Geometry check sheet. Reference: the model listing, model coordinates, mm. A direction names the side the tool comes from. Coordinates: 2 decimals unless noted, no trailing zeros. Write each loop counter-clockwise with the first axis right and the second up, starting at its lowest first coordinate (ties: lowest second). Pieces come first, ordered by that corner, then holes. Notation, with made-up numbers: (70, -16.75) -> (120, -16.75) arc R27 cw to (120, 9.25) -> close; hole circle Ø8 at (75, 56). An arc over 180 degrees is marked (long way). One line per question, with ' | ' between items.
```python
from build123d import *

# Parameters (mm, degrees)
EXTRUDE_1_DEPTH                = 4
CUT_EXTRUDE_1_DEPTH            = 105.27847333
CUT_EXTRUDE_1_DEPTH_BACK       = 105.27847333
SKETCH_2_R                     = 2
SKETCH_2_W                     = 4
SKETCH_2_H                     = 16
CHAMFER_1_SIZE                 = 1
CUT_EXTRUDE_2_DEPTH            = 105.27847333
CUT_EXTRUDE_2_DEPTH_BACK       = 105.27847333
SKETCH_6_W                     = 20
SKETCH_6_H                     = 5
EXTRUDE_2_DEPTH                = 25
CHAMFER_2_SIZE                 = 1
EXTRUDE_START                  = -5
EXTRUDE_3_DEPTH                = 5
SKETCH_8_R                     = 6
EXTRUDE_4_DEPTH                = 5
CHAMFER_3_SIZE                 = 1
SKETCH_9_R                     = 4
EXTRUDE_5_DEPTH                = 5
CUT_EXTRUDE_START              = -10
SKETCH_10_R                    = 2
CUT_EXTRUDE_3_DEPTH            = 120.608393839
HOLE_WIZARD_1_4_0_15748031_1_D = 3.999999874
SKETCH_13_R                    = 1.5
CUT_EXTRUDE_4_DEPTH            = 109.434311913
SKETCH_14_R                    = 2
CUT_EXTRUDE_5_DEPTH            = 109.434311913
CUT_EXTRUDE_START_2            = 10
SKETCH_15_R                    = 4
CUT_EXTRUDE_6_DEPTH            = 10
CHAMFER_4_SIZE                 = 2
CHAMFER_5_SIZE                 = 1
SKETCH_16_W                    = 18
SKETCH_16_H                    = 4
CUT_EXTRUDE_7_DEPTH            = 109.434311913
SKETCH_17_R                    = 1.5
CUT_EXTRUDE_8_DEPTH            = 3


with BuildPart() as part:
    # 草图1 → 凸台-拉伸1 (new body)
    with BuildSketch(Plane(origin=(0, 0, 0), x_dir=(1, 0, 0), z_dir=(0, 1, 0))):
        Polygon((0, -34), (0, 34), (17, 47), (32, 47), (32, 34), (55, 34), (55, 47), (61, 47), (63, 45), (93, 45), (93, -45), (63, -45), (61, -47), (55, -47), (55, -34), (32, -34), (32, -47), (17, -47), align=None)
    extrude(amount=EXTRUDE_1_DEPTH)

    # 草图2 → 切除-拉伸1 (cut, two sides: drawn at the far end of the back side and taken through both)
    with BuildSketch(Plane(origin=(0, 4, 0), x_dir=(1, 0, 0), z_dir=(0, 1, 0)).offset(-CUT_EXTRUDE_1_DEPTH_BACK)):
        with Locations(Location((13, 10, 0), (0, 0, 270))):
            Circle(SKETCH_2_R)
        with Locations(Location((13, -10, 0), (0, 0, 90))):
            Circle(SKETCH_2_R)
        with Locations((6, 0)):
            Rectangle(SKETCH_2_W, SKETCH_2_H)
        Polygon((4, 12), (4, 26), (17, 36.408329997), (17, 33.205766921), (8, 26), (8, 12), align=None)
        Polygon((8, -26), (8, -12), (4, -12), (4, -26), (17, -36.408329997), (17, -33.205766921), align=None)
    extrude(amount=CUT_EXTRUDE_1_DEPTH + CUT_EXTRUDE_1_DEPTH_BACK, mode=Mode.SUBTRACT)

    # 倒角1
    chamfer_1_edges = [part.edges().sort_by_distance(p)[0] for p in [
        (8.5, 4, 40.5),
        (24.5, 4, 47),
        (8.5, 4, -40.5),
        (24.5, 4, -47),
        (0, 4, 0),
    ]]
    chamfer(chamfer_1_edges, length=CHAMFER_1_SIZE)

    # 草图3 → 切除-拉伸2 (cut, two sides: drawn at the far end of the back side and taken through both)
    with BuildSketch(Plane(origin=(0, 4, 0), x_dir=(1, 0, 0), z_dir=(0, 1, 0)).offset(-CUT_EXTRUDE_2_DEPTH_BACK)):
        Polygon((93, 22), (33, 22), (21, 10), (21, -10), (33, -22), (93, -22), align=None)
    extrude(amount=CUT_EXTRUDE_2_DEPTH + CUT_EXTRUDE_2_DEPTH_BACK, mode=Mode.SUBTRACT)

    # 草图6 → 凸台-拉伸2 (add)
    with BuildSketch(Plane(origin=(0, 4, 0), x_dir=(1, 0, 0), z_dir=(0, 1, 0))):
        with BuildLine():
            Line((21, 10), (21, 15))
            ThreePointArc((21, 15), (15, 21), (21, 27))
            Line((21, 27), (33, 27))
            Line((33, 27), (33, 22))
            Line((33, 22), (21, 10))
        make_face()
        with Locations((83, 24.5)):
            Rectangle(SKETCH_6_W, SKETCH_6_H)
    extrude_2 = extrude(amount=EXTRUDE_2_DEPTH)

    # 镜向1: 凸台-拉伸2 across plane
    add(extrude_2.mirror(Plane.XY))

    # 倒角2
    chamfer_2_edges = [part.edges().sort_by_distance(p)[0] for p in [
        (83, 4, -27),
        (73, 4, -24.5),
        (83, 4, 27),
        (73, 4, 24.5),
    ]]
    chamfer(chamfer_2_edges, length=CHAMFER_2_SIZE)

    # 草图7 → 凸台-拉伸3 (add)
    with BuildSketch(Plane(origin=(0, 29, 0), x_dir=(1, 0, 0), z_dir=(0, 1, 0)).offset(EXTRUDE_START)):
        with BuildLine():
            Line((93, 22), (93, 27))
            Line((93, 27), (73, 27))
            Line((73, 27), (73, 21))
            Line((73, 21), (53, 21))
            Line((53, 21), (53, 27))
            Line((53, 27), (33, 27))
            Line((33, 27), (21, 27))
            ThreePointArc((21, 27), (15, 21), (21, 15))
            Line((21, 15), (21, 10))
            Line((21, 10), (21, -10))
            Line((21, -10), (21, -15))
            ThreePointArc((21, -15), (15, -21), (21, -27))
            Line((21, -27), (33, -27))
            Line((33, -27), (53, -27))
            Line((53, -27), (53, -21))
            Line((53, -21), (73, -21))
            Line((73, -21), (73, -27))
            Line((73, -27), (93, -27))
            Line((93, -27), (93, -22))
            Line((93, -22), (93, 22))
        make_face()
    extrude(amount=EXTRUDE_3_DEPTH)

    # 草图8 → 凸台-拉伸4 (add)
    with BuildSketch(Plane(origin=(0, 29, 0), x_dir=(1, 0, 0), z_dir=(0, 1, 0))):
        with Locations(Location((21, 21, 0), (0, 0, 270))):
            Circle(SKETCH_8_R)
        with Locations(Location((21, -21, 0), (0, 0, 270))):
            Circle(SKETCH_8_R)
    extrude(amount=EXTRUDE_4_DEPTH)

    # 倒角3
    chamfer_3_edges = [part.edges().sort_by_distance(p)[0] for p in [
        (21, 34, -27),
        (21, 34, 15),
    ]]
    chamfer(chamfer_3_edges, length=CHAMFER_3_SIZE)

    # 草图9 → 凸台-拉伸5 (add)
    with BuildSketch(Plane(origin=(0, 29, 0), x_dir=(1, 0, 0), z_dir=(0, 1, 0))):
        with Locations(Location((83, 21, 0), (0, 0, 270))):
            Circle(SKETCH_9_R)
    extrude_5 = extrude(amount=EXTRUDE_5_DEPTH)

    # 草图10 → 切除-拉伸3 (cut)
    with BuildSketch(Plane(origin=(0, 34, 0), x_dir=(1, 0, 0), z_dir=(0, 1, 0)).offset(CUT_EXTRUDE_START)):
        with Locations(Location((83, 21, 0), (0, 0, 270))):
            Circle(SKETCH_10_R)
    cut_extrude_3 = extrude(amount=CUT_EXTRUDE_3_DEPTH, mode=Mode.SUBTRACT)

    # 镜向2: 凸台-拉伸5, 切除-拉伸3 across plane
    add(extrude_5.mirror(Plane.XY))
    add(cut_extrude_3.mirror(Plane.XY), mode=Mode.SUBTRACT)

    # 1/4 (0.15748031) 直径孔1 (through all)
    with Locations(Plane(origin=(21, 34, -21), x_dir=(0, 0, 1), z_dir=(0, 1, 0))):
        with Locations((0, 0)):
            hole_wizard_1_4_0_15748031_1 = Hole(HOLE_WIZARD_1_4_0_15748031_1_D / 2)

    # 镜向3: 1/4 (0.15748031) 直径孔1 across plane
    add(hole_wizard_1_4_0_15748031_1.mirror(Plane.XY), mode=Mode.SUBTRACT)

    # 草图13 → 切除-拉伸4 (cut, symmetric)
    with BuildSketch(Plane(origin=(0, 4, 0), x_dir=(1, 0, 0), z_dir=(0, 1, 0))):
        with Locations(Location((29, 40, 0), (0, 0, 270))):
            Circle(SKETCH_13_R)
        with Locations(Location((58, 40, 0), (0, 0, 270))):
            Circle(SKETCH_13_R)
    cut_extrude_4 = extrude(amount=CUT_EXTRUDE_4_DEPTH, both=True, mode=Mode.SUBTRACT)

    # 镜向4: 切除-拉伸4 across plane
    add(cut_extrude_4.mirror(Plane.XY), mode=Mode.SUBTRACT)

    # 草图14 → 切除-拉伸5 (cut, symmetric)
    with BuildSketch(Plane(origin=(0, 4, 0), x_dir=(1, 0, 0), z_dir=(0, 1, 0))):
        with Locations(Location((63, 27, 0), (0, 0, 270))):
            Circle(SKETCH_14_R)
    cut_extrude_5 = extrude(amount=CUT_EXTRUDE_5_DEPTH, both=True, mode=Mode.SUBTRACT)

    # 镜向5: 切除-拉伸5 across plane
    add(cut_extrude_5.mirror(Plane.XY), mode=Mode.SUBTRACT)

    # 草图15 → 切除-拉伸6 (cut)
    with BuildSketch(Plane.XZ.offset(-24).offset(CUT_EXTRUDE_START_2)):
        with Locations(Location((83, 21, 0), (0, 0, 270))):
            Circle(SKETCH_15_R)
        with Locations(Location((83, -21, 0), (0, 0, 90))):
            Circle(SKETCH_15_R)
    extrude(amount=-CUT_EXTRUDE_6_DEPTH, mode=Mode.SUBTRACT)

    # 倒角4
    chamfer_4_edges = [part.edges().sort_by_distance(p)[0] for p in [
        (83, 24, -23),
        (83, 24, 23),
    ]]
    chamfer(chamfer_4_edges, length=CHAMFER_4_SIZE - 0.0001)  # a hair under: the kernel refuses the full size

    # 倒角5
    chamfer_5_edges = [part.edges().sort_by_distance(p)[0] for p in [
        (83, 34, -25),
        (83, 34, 25),
    ]]
    chamfer(chamfer_5_edges, length=CHAMFER_5_SIZE)

    # 草图16 → 切除-拉伸7 (cut, through all)
    with BuildSketch(Plane(origin=(0, 4, 0), x_dir=(1, 0, 0), z_dir=(0, 1, 0))):
        with Locations((84, 39)):
            Rectangle(SKETCH_16_W, SKETCH_16_H)
    cut_extrude_7 = extrude(amount=-CUT_EXTRUDE_7_DEPTH, mode=Mode.SUBTRACT)

    # 镜向6: 切除-拉伸7 across plane
    add(cut_extrude_7.mirror(Plane.XY), mode=Mode.SUBTRACT)

    # 草图17 → 切除-拉伸8 (cut)
    with BuildSketch(Plane(origin=(93, 0, 0), x_dir=(0, 0, -1), z_dir=(1, 0, 0))):
        with Locations((24.5, 4)):
            Circle(SKETCH_17_R)
    cut_extrude_8 = extrude(amount=-CUT_EXTRUDE_8_DEPTH, mode=Mode.SUBTRACT)

    # 镜向7: 切除-拉伸8 across plane
    add(cut_extrude_8.mirror(Plane.XY), mode=Mode.SUBTRACT)


solid = part.part
```
(1) Cross-section at A-A (y = 8). Record the cut outline in (x, z), plus the area to 3 significant figures.
Answers below:
outline: (21, -27) -> (33, -27) -> (33, -22) -> (21, -10) -> (21, -15) arc R6 ccw to start; (21, 10) -> (33, 22) -> (33, 27) -> (21, 27) arc R6 ccw to (21, 15) -> close; (73, -27) -> (93, -27) -> (93, -22) -> (73, -22) -> close; (73, 22) -> (93, 22) -> (93, 27) -> (73, 27) -> close; hole circle Ø4 at (21, -21); hole circle Ø4 at (21, 21) | area: 552 mm²
(2) Depth check by flat-ended pin: P1, Ø8, axis at x = 10, y = 4, coming from the -Z side; P2, Ø4.5, axis at x = 85, y = 3, coming from the -Z side; P3, Ø1.2, axis at y = 2.5, z = -3.5, coming from the +X side. Enter the tip coordinate at first touch or a pass-through.
Answers below:
P1: stops at z = -44.61 | P2: stops at z = -45 | P3: stops at x = 21
(3) Draft check along X on faces 4 (the face through (82, 34, -19)), 5 (the face through (6, 2, 8)), 6 (the face through (93, 2, 43)). Enter one of: pulls with the +X half, pulls with the -X half, needs draft (parallel to the pull), parting line crosses it, or undercut.
Answers below:
face 4: needs draft | face 5: undercut | face 6: pulls with the +X half
(4) Material ranges on line 1 (X direction, y = 30.5, z = -21); line 2 (X direction, y = 2, z = 40); line 3 (X direction, y = 1.7, z = 10), recorded low to high.
Answers below:
line 1: x = 15 to 19, 23 to 27, 79 to 81, 85 to 87 | line 2: x = 7.85 to 27.5, 30.5 to 32, 55 to 56.5, 59.5 to 75 | line 3: x = 0 to 11, 15 to 21
(5) Cross-section at B-B (x = 58). Record the cut outline in (y, z), plus the area to 3 significant figures.
Answers below:
outline: (0, -47) -> (4, -47) -> (4, -41.5) -> (0, -41.5) -> close; (0, -38.5) -> (4, -38.5) -> (4, -22) -> (0, -22) -> close; (0, 22) -> (4, 22) -> (4, 38.5) -> (0, 38.5) -> close; (0, 41.5) -> (4, 41.5) -> (4, 47) -> (0, 47) -> close; (24, -21) -> (29, -21) -> (29, 21) -> (24, 21) -> close | area: 386 mm²
(6) Tool access check on faces 1 (the face through (63, 26, -21)), 2 (the face through (78, 2, 45)), 3 (the face through (15.677, 18.297, -18.231)). Record the directions out of +Z, -Z, +X, -X, +Y, -Y that give a thin tool (end or side, any length) a straight path to the whole face; none if there is none.
Answers below:
face 1: -Z, +Y, -Y | face 2: +Z, +X, +Y, -Y | face 3: +Y
